from build123d import *

# Parameters (mm, degrees)
F0_W        = 20
F0_H        = 20
F1_DEPTH    = 20
F2_R        = 5
F3_R        = 1
F4_T1_DEPTH = 20.75
F5_T1_DEPTH = 20.75


# Not quite as in the source:
# - a fillet or chamfer that OpenCascade refuses, or shapes differently, is made with other operations: its cross-section is extruded or revolved along the edge and cut away or added


with BuildPart() as f1:
    # F0 (on Front) → F1 (new body)
    with BuildSketch(Plane.XZ):
        with Locations((-5, 50)):
            Rectangle(F0_W, F0_H)
    extrude(amount=F1_DEPTH)

    # F2
    f2_edges = [f1.edges().sort_by_distance(p)[0] for p in [
        (-15, -10, 40),
        (5, -10, 40),
        (-5, 0, 40),
        (-5, -20, 40),
    ]]
    fillet(f2_edges, radius=F2_R)

    # F3
    f3_edges = [f1.edges().sort_by_distance(p)[0] for p in [
        (5, -10, 60),
        (-15, -10, 60),
        (-5, 0, 60),
        (-5, -20, 60),
    ]]
    fillet(f3_edges, radius=F3_R)

    # F4: fillet of radius 1 on 4 edges, made by hand

    # F4_s2 → F4_t1 (cut)
    with BuildSketch(Plane.XY.offset(40.75)):
        with BuildLine():
            ThreePointArc((4, 0), (4.7071067812, -0.2928932188), (5, -1))
            Line((5, -1), (5, 0))
            Line((5, 0), (4, 0))
        make_face()
        with BuildLine():
            ThreePointArc((4, -20), (4.7071067812, -19.7071067812), (5, -19))
            Line((5, -19), (5, -20))
            Line((5, -20), (4, -20))
        make_face()
    extrude(amount=F4_T1_DEPTH, mode=Mode.SUBTRACT)

    # F5: fillet of radius 1 on 4 edges, made by hand

    # F5_s2 → F5_t1 (cut)
    with BuildSketch(Plane.XY.offset(40.75)):
        with BuildLine():
            ThreePointArc((-15, -1), (-14.7071067812, -0.2928932188), (-14, 0))
            Line((-14, 0), (-15, 0))
            Line((-15, 0), (-15, -1))
        make_face()
        with BuildLine():
            ThreePointArc((-15, -19), (-14.7071067812, -19.7071067812), (-14, -20))
            Line((-14, -20), (-15, -20))
            Line((-15, -20), (-15, -19))
        make_face()
    extrude(amount=F5_T1_DEPTH, mode=Mode.SUBTRACT)


solid = f1.part
Model file for the job. Use its own axes, mm. Give positions to 0.01 mm unless a question says otherwise; leave off trailing zeros. Loops run counter-clockwise (first coordinate to the right, second up) from the corner with the lowest first, then second, coordinate; pieces in that order, holes last. Notation, with made-up numbers: (28.25, 10) -> (84.25, 10) arc R17 ccw to (84.25, 31) -> close; hole circle Ø10 at (48, 50.25). An arc over 180 degrees is marked (long way). Use a Markdown table: item, result. Add a question column.
(1) Slice it at B-B on x = -2.75. List the corners of the cut face in (y, z).
(2) Slice it at A-A on y = -9.5. List the corners of the cut face in (x, z).
(3) Wall check: line 1 along Z through (x, y) = (0.25, -7.75); line 2 along X through (y, z) = (-6.75, 42); line 3 along Y through (x, z) = (2.25, 41). Give the ranges that are in metal, low to high.
(4) Slice it at C-C on z = 42.5. List the corners of the cut face in (x, y), and give its area (3 significant figures).
Filled sheet:
| question | item | result |
|---|---|---|
| 1 | outline | (-20, 45) arc R5 ccw to (-15, 40) -> (-5, 40) arc R5 ccw to (0, 45) -> (0, 59) arc R1 ccw to (-1, 60) -> (-19, 60) arc R1 ccw to (-20, 59) -> close |
| 2 | outline | (-15, 45) arc R5 ccw to (-10, 40) -> (0, 40) arc R5 ccw to (5, 45) -> (5, 59) arc R1 ccw to (4, 60) -> (-14, 60) arc R1 ccw to (-15, 59) -> close |
| 3 | line 1 | 40.01 to 60 |
| 3 | line 2 | -14 to 4 |
| 3 | line 3 | -18 to -2 |
| 4 | outline | (-14.33, -19.33) -> (4.33, -19.33) -> (4.33, -0.67) -> (-14.33, -0.67) -> close |
| 4 | area | 348 mm2 |
